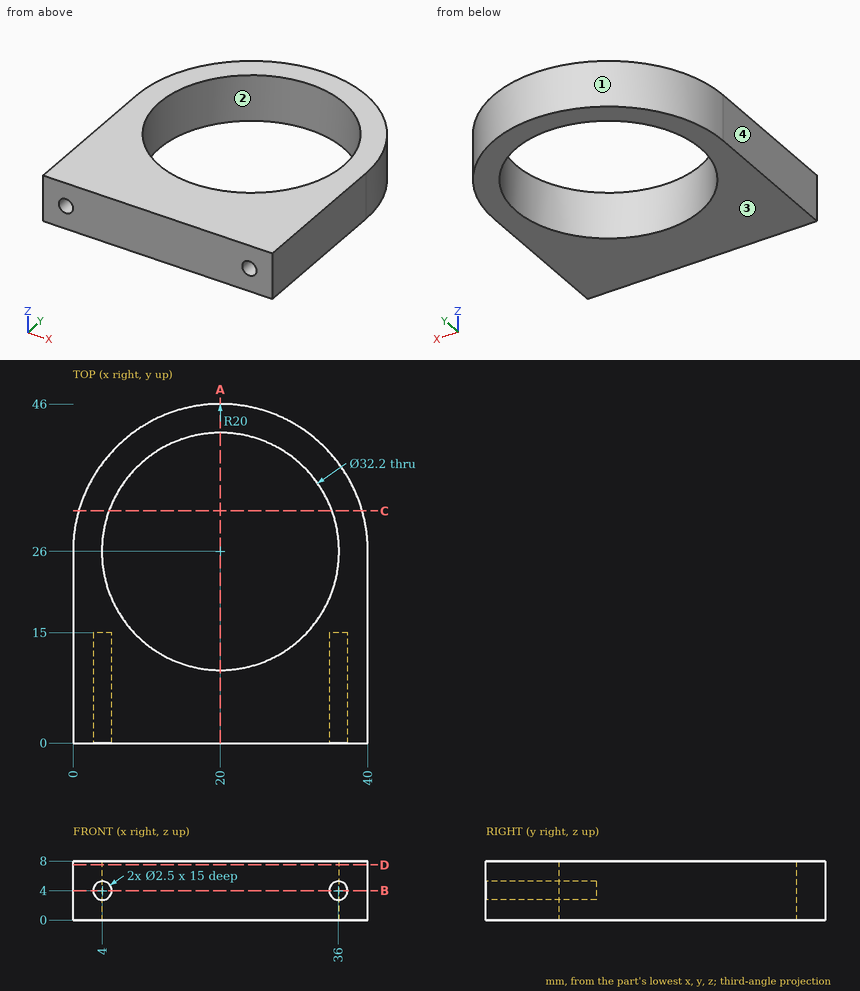
Could you check a few things on this drawing? It's one solid part, dimensions in mm from its lowest x, y, z. Give positions to 0.01 mm unless a question says otherwise; leave off trailing zeros. Order: outer loops, then holes, each group sorted by start corner. A loop starts at its lowest first (then second) coordinate and runs counter-clockwise, first axis right, second up.
1. Suppose I cut it at C-C (y = 31.5). Write out the boundary of the cut face in (x, z), plus the area to 3 significant figures.
Answers below:
outline: (0.77, 0) - (4.87, 0) - (4.87, 8) - (0.77, 8) - close; (35.13, 0) - (39.23, 0) - (39.23, 8) - (35.13, 8) - close
area: 65.6 mm2
2. For pin 1 (1 mm diameter, centred on y = 35.5, z = 5, fed in from -X); pin 2 (4 mm diameter, centred on x = 36, z = 4, fed in from +Y); pin 3 (0.8 mm diameter, centred on x = 36.5, z = 4, fed in from -Y), each with a flat end and sliding along its axis, tell me the tip position at first contact or that it passes through.
Answers below:
pin 1: stops at x = 2.14
pin 2: stops at y = 40.28
pin 3: stops at y = 15
3. Suppose I cut it at A-A (x = 20). Write out the boundary of the cut face in (y, z).
Answers below:
outline: (0, 0) - (9.9, 0) - (9.9, 8) - (0, 8) - close; (42.1, 0) - (46, 0) - (46, 8) - (42.1, 8) - close
4. I need wall thicknesses on L1, parallel to X at y = 26.5, z = 3.75; L2, parallel to Z at x = 4, y = 10.75; L3, parallel to Y at x = 20, z = 4.25. Which ranges of each line are inside material? Lowest first, please.
Answers below:
L1: x = 0.01 to 3.91, 36.09 to 39.99
L2: z = 0 to 2.75, 5.25 to 8
L3: y = 0 to 9.9, 42.1 to 46
5. Suppose I cut it at B-B (z = 4). Write out the boundary of the cut face in (x, y).
Answers below:
outline: (0, 0) - (2.75, 0) - (2.75, 15) - (5.25, 15) - (5.25, 0) - (34.75, 0) - (34.75, 15) - (37.25, 15) - (37.25, 0) - (40, 0) - (40, 26) arc R20 ccw to (0, 26) - close; hole circle Ø32.2 at (20, 26)
6. Suppose I cut it at D-D (z = 7.5). Write out the boundary of the cut face in (x, y).
Answers below:
outline: (0, 0) - (40, 0) - (40, 26) arc R20 ccw to (0, 26) - close; hole circle Ø32.2 at (20, 26)
7. Thinking about a two-plate mould opening in X: for the marked faces 1, 2, 3 and 4, which applies, +X half, -X half, draft (parallel to the pull), parting line (faces both ways), or undercut?
Answers below:
face 1: parting line
face 2: undercut
face 3: draft
face 4: -X half
